Check sheet for the modelled part. Datum: model origin and axes. Units: mm. Face numbers are marked on the shaded views. A direction names the side the tool comes from. Give positions to 0.01 mm unless a question says otherwise; leave off trailing zeros. Loops run counter-clockwise (first coordinate to the right, second up) from the corner with the lowest first, then second, coordinate; pieces in that order, holes last. Notation, with made-up numbers: (45, -15) -> (92, -15) arc R10 ccw to (92, 2) -> close; hole circle Ø1 at (0.5, 74). An arc over 180 degrees is marked (long way). Write each question's results on one line, items separated by ' | '. Start each with the question number.
1. Cross-section at A-A on x = -27. Record the boundary of the cut face in (y, z), and give its area (3 significant figures).
2. Material ranges on L1, parallel to X at y = 3.5, z = 12.5; L2, parallel to X at y = 5, z = 14.5; L3, parallel to Z at x = 14, y = 1.25, recorded low to high. Write a range as from..to.
3. Gauge pin test, flat ends, axial feed: pin 1 Ø1.8 at (x, z) = (-14.82, -8.56) entering from +Y; pin 2 Ø1.3 at (y, z) = (2.5, 0) entering from -X; pin 3 Ø2 at (x, y) = (8.5, 5) entering from -Z. Record the tip position at first contact, or that the pin passes through.
4. Cross-section at D-D on z = -35. Record the boundary of the cut face in (x, y), and give its area (3 significant figures).
5. Cross-section at B-B on y = 1.25. Count the separate pieces of the cut face and the enclosed holes in it, and give its area (3 significant figures).
6. Cross-section at C-C on z = -22. Record the boundary of the cut face in (x, y), and give its area (3 significant figures).
7. Mould release check, pull along Z, two halves, no side actions. Record for the marked faces 1, 2 and 3: +Z half, -Z half, draft (parallel to the pull), parting line (faces both ways), or undercut.
8. Tool access check on the marked faces 4, 5 and 6. Record the directions out of +Z, -Z, +X, -X, +Y, -Y that give a thin tool (end or side, any length) a straight path to the whole face; none if there is none.
from build123d import *

# Parameters (mm, degrees)
SKETCH1_R           = 41.91
BOSS_EXTRUDE1_DEPTH = 6.35
CUT_EXTRUDE1_DEPTH  = 7.35
SKETCH3_R           = 1.016
CUT_EXTRUDE2_DEPTH  = 7.35


with BuildPart() as part:
    # Sketch1 → Boss-Extrude1 (new body)
    with BuildSketch(Plane(origin=(0, 0, 0), x_dir=(1, 0, 0), z_dir=(0, 1, 0))):
        Circle(SKETCH1_R)
    extrude(amount=BOSS_EXTRUDE1_DEPTH)

    # Sketch2 → Cut-Extrude1 (cut, through all)
    with BuildSketch(Plane(origin=(0, 6.35, 0), x_dir=(1, 0, 0), z_dir=(0, 1, 0))):
        with BuildLine():
            Line((-1.440684381, 5.03409922), (-11.531101351, 40.292453408))
            ThreePointArc((-11.531101351, 40.292453408), (-20.955, 36.295124673), (-29.128737556, 30.132453408))
            Line((-29.128737556, 30.132453408), (-3.639315619, 3.764718883))
            Line((-3.639315619, 3.764718883), (-1.440684381, 5.03409922))
        make_face()
        with BuildLine():
            Line((3.639315619, 3.764718883), (29.128737556, 30.132453408))
            ThreePointArc((29.128737556, 30.132453408), (20.955, 36.295124673), (11.531101351, 40.292453408))
            Line((11.531101351, 40.292453408), (1.440684381, 5.03409922))
            Line((1.440684381, 5.03409922), (3.639315619, 3.764718883))
        make_face()
        with BuildLine():
            Line((5.08, -1.269380337), (40.659838908, -10.16))
            ThreePointArc((40.659838908, -10.16), (41.596285583, -5.118312778), (41.91, 0))
            ThreePointArc((41.91, 0), (41.596285583, 5.118312778), (40.659838908, 10.16))
            Line((40.659838908, 10.16), (5.08, 1.269380337))
            Line((5.08, 1.269380337), (5.08, -1.269380337))
        make_face()
        with BuildLine():
            ThreePointArc((11.531101351, -40.292453408), (20.955, -36.295124673), (29.128737556, -30.132453408))
            Line((29.128737556, -30.132453408), (3.639315619, -3.764718883))
            Line((3.639315619, -3.764718883), (1.440684381, -5.03409922))
            Line((1.440684381, -5.03409922), (11.531101351, -40.292453408))
        make_face()
        with BuildLine():
            ThreePointArc((-29.128737556, -30.132453408), (-20.955, -36.295124673), (-11.531101351, -40.292453408))
            Line((-11.531101351, -40.292453408), (-1.440684381, -5.03409922))
            Line((-1.440684381, -5.03409922), (-3.639315619, -3.764718883))
            Line((-3.639315619, -3.764718883), (-29.128737556, -30.132453408))
        make_face()
        with BuildLine():
            ThreePointArc((-40.659838908, 10.16), (-41.91, 0), (-40.659838908, -10.16))
            Line((-40.659838908, -10.16), (-5.08, -1.269380337))
            Line((-5.08, -1.269380337), (-5.08, 1.269380337))
            Line((-5.08, 1.269380337), (-40.659838908, 10.16))
        make_face()
    extrude(amount=-CUT_EXTRUDE1_DEPTH, mode=Mode.SUBTRACT)

    # Sketch3 → Cut-Extrude2 (cut, through all)
    with BuildSketch(Plane(origin=(0, 6.35, 0), x_dir=(1, 0, 0), z_dir=(0, 1, 0))):
        with Locations((17.417935934, -10.05625)):
            Circle(SKETCH3_R)
        with Locations((-7.05625, -12.221783511)):
            Circle(SKETCH3_R)
        with Locations((-8.55625, -14.819859722)):
            Circle(SKETCH3_R)
        with Locations((-10.05625, -17.417935934)):
            Circle(SKETCH3_R)
        with Locations((-9.6237073, 5.55625)):
            Circle(SKETCH3_R)
        with Locations((5.55625, 9.6237073)):
            Circle(SKETCH3_R)
        with Locations((9.6237073, -5.55625)):
            Circle(SKETCH3_R)
        with Locations((-5.55625, -9.6237073)):
            Circle(SKETCH3_R)
        with Locations((-14.819859722, 8.55625)):
            Circle(SKETCH3_R)
        with Locations((-17.417935934, 10.05625)):
            Circle(SKETCH3_R)
        with Locations((-12.221783511, 7.05625)):
            Circle(SKETCH3_R)
        with Locations((7.05625, 12.221783511)):
            Circle(SKETCH3_R)
        with Locations((8.55625, 14.819859722)):
            Circle(SKETCH3_R)
        with Locations((10.05625, 17.417935934)):
            Circle(SKETCH3_R)
        with Locations((12.221783511, -7.05625)):
            Circle(SKETCH3_R)
        with Locations((14.819859722, -8.55625)):
            Circle(SKETCH3_R)
    extrude(amount=-CUT_EXTRUDE2_DEPTH, mode=Mode.SUBTRACT)


solid = part.part
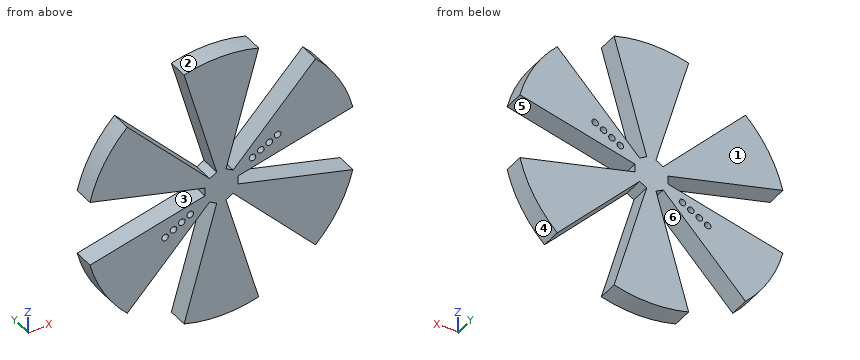
Geometry says:
1) outline: (0, -27.93) -> (6.35, -27.93) -> (6.35, -6.75) -> (0, -6.75) -> close; (0, 6.75) -> (6.35, 6.75) -> (6.35, 27.93) -> (0, 27.93) -> close | area: 269 mm^2
2) L1: -40..-12.08, -3.58..3.58, 12.08..40 | L2: -39.32..-14.02, -4.15..4.15, 14.02..39.32 | L3: -14.48..-3.5, 3.5..7.96, 9.16..14.48
3) pin 1: through | pin 2: x = -5.08 | pin 3: z = -41.23
4) outline: (-10.02, 0) -> (10.02, 0) -> (10.02, 6.35) -> (-10.02, 6.35) -> close | area: 127 mm^2
5) separate pieces: 1 | enclosed holes: 8 | area: 2,950 mm^2
6) outline: (-35.67, 0) -> (-21.27, 0) -> (-21.27, 6.35) -> (-35.67, 6.35) -> close; (-6.3, 0) -> (6.3, 0) -> (6.3, 6.35) -> (-6.3, 6.35) -> close; (21.27, 0) -> (35.67, 0) -> (35.67, 6.35) -> (21.27, 6.35) -> close | area: 263 mm^2
7) face 1: draft | face 2: +Z half | face 3: undercut
8) face 4: -Z, +X, +Y, -Y | face 5: +X, +Y, -Y | face 6: +Y, -Y
